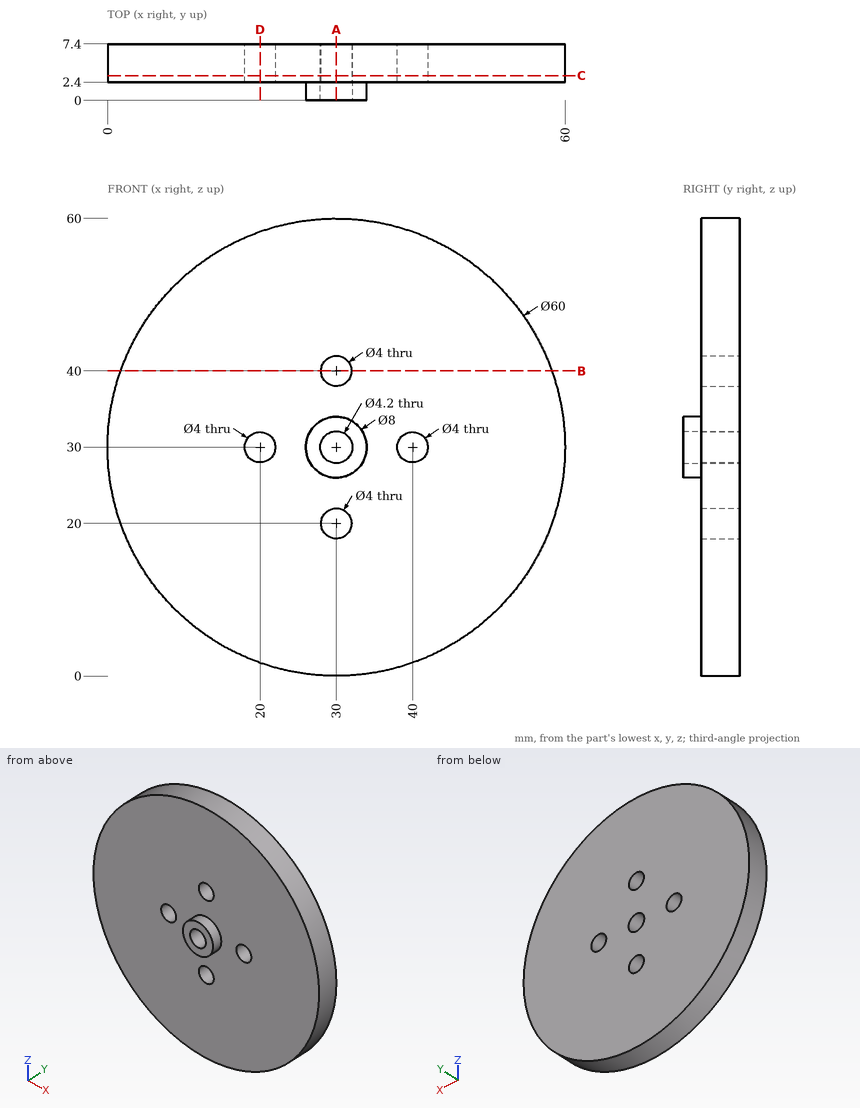
For this review, use the dimensioned drawing (mm, ordinates from the lowest corner) and the shaded views. Round coordinates to 2 decimals unless told otherwise and drop trailing zeros. Order: outer loops, then holes, each group sorted by start corner. A loop starts at its lowest first (then second) coordinate and runs counter-clockwise, first axis right, second up.
1) Consider section C-C (y = 3.25). State the section outline as (x, z) points.
The answers:
outline: circle Ø60 at (30, 30); hole circle Ø4 at (20, 30); hole circle Ø4.2 at (30, 30); hole circle Ø4 at (30, 20); hole circle Ø4 at (30, 40); hole circle Ø4 at (40, 30)
2) Clearance check with flat-ended pins moving along their axes: pin 1 Ø2.5 at (x, z) = (20, 30) entering from +Y; pin 2 Ø6.5 at (x, z) = (30, 40) entering from -Y; pin 3 Ø4 at (x, y) = (36.5, 2) entering from +Z. State where each tip first meets the part, or that it passes through.
The answers:
pin 1: passes through
pin 2: stops at y = 2.4
pin 3: stops at z = 59.65
3) Consider section A-A (x = 30). State the section outline as (y, z) points, plus the area to 3 significant figures.
The answers:
outline: (0, 26) - (2.4, 26) - (2.4, 22) - (7.4, 22) - (7.4, 27.9) - (0, 27.9) - close; (0, 32.1) - (7.4, 32.1) - (7.4, 38) - (2.4, 38) - (2.4, 34) - (0, 34) - close; (2.4, 0) - (7.4, 0) - (7.4, 18) - (2.4, 18) - close; (2.4, 42) - (7.4, 42) - (7.4, 60) - (2.4, 60) - close
area: 248 mm2
4) For L1, parallel to X at y = 4.15, z = 30; L2, parallel to Y at x = 37, z = 54, list the stretches that pass through material, from the lowest coordinate up.
The answers:
L1: x = 0 to 18, 22 to 27.9, 32.1 to 38, 42 to 60
L2: y = 2.4 to 7.4
5) Consider section B-B (z = 40). State the section outline as (x, y) points, plus the area to 3 significant figures.
The answers:
outline: (1.72, 2.4) - (28, 2.4) - (28, 7.4) - (1.72, 7.4) - close; (32, 2.4) - (58.28, 2.4) - (58.28, 7.4) - (32, 7.4) - close
area: 263 mm2
6) Consider section D-D (x = 20). State the section outline as (y, z) points.
The answers:
outline: (2.4, 1.72) - (7.4, 1.72) - (7.4, 28) - (2.4, 28) - close; (2.4, 32) - (7.4, 32) - (7.4, 58.28) - (2.4, 58.28) - close
